from build123d import *

# Parameters (mm, degrees)
SKETCH_1_W          = 8
SKETCH_1_H          = 5
EXTRUDE_1_DEPTH     = 4
SKETCH_2_W          = 2
SKETCH_2_H          = 5
CUT_EXTRUDE_1_DEPTH = 3
SKETCH_3_R          = 1.65
CUT_EXTRUDE_2_DEPTH = 5


with BuildPart() as part:
    # Эскиз1 → Бобышка-Вытянуть1 (new body)
    with BuildSketch(Plane.XY):
        Rectangle(SKETCH_1_W, SKETCH_1_H)
    extrude(amount=EXTRUDE_1_DEPTH)

    # Эскиз2 → Вырез-Вытянуть1 (cut)
    with BuildSketch(Plane(origin=(4, 0, 0), x_dir=(0, 0, -1), z_dir=(1, 0, 0))):
        with Locations((-3, 0)):
            Rectangle(SKETCH_2_W, SKETCH_2_H)
    extrude(amount=-CUT_EXTRUDE_1_DEPTH, mode=Mode.SUBTRACT)

    # Эскиз3 → Вырез-Вытянуть2 (cut)
    with BuildSketch(Plane.XY.offset(4)):
        with Locations((-1.5, 0)):
            Circle(SKETCH_3_R)
    extrude(amount=-CUT_EXTRUDE_2_DEPTH, mode=Mode.SUBTRACT)


solid = part.part
Model file for the job. Use its own axes, mm. A direction names the side the tool comes from. Give positions to 0.01 mm unless a question says otherwise; leave off trailing zeros. Write each loop counter-clockwise with the first axis right and the second up, starting at its lowest first coordinate (ties: lowest second). Pieces come first, ordered by that corner, then holes. Notation, with made-up numbers: (49, -19) -> (79, -19) arc R27 cw to (79, 1) -> close; hole circle Ø8 at (-1, -10.75). An arc over 180 degrees is marked (long way). Write item = value, one per line.
(1) Mould opens along Y. For faces 3 (the face through (4, 0, 1)), 4 (the face through (0.074, 0.496, 2.028)), 5 (the face through (-1, -2.5, 2)), 6 (the face through (-1, 2.5, 2)) say: released by +Y, released by -Y, zero draft, split by the parting line, or undercut.
Determined:
face_3 = zero draft
face_4 = undercut
face_5 = released by -Y
face_6 = released by +Y
(2) Slice it at D-D, the plane y = -2.05. Give the cut face in (x, z), then the cut area to 3 significant figures.
Determined:
outline = (-4, 0) -> (4, 0) -> (4, 2) -> (1, 2) -> (1, 4) -> (-4, 4) -> close
area = 26.0 mm2
(3) Slice it at C-C, the plane z = 0.4. Give the cut face in (x, y), then the cut area to 3 significant figures.
Determined:
outline = (-4, -2.5) -> (4, -2.5) -> (4, 2.5) -> (-4, 2.5) -> close; hole circle Ø3.3 at (-1.5, 0)
area = 31.4 mm2
(4) Slice it at B-B, the plane x = -1.5. Give the cut face in (y, z).
Determined:
outline = (-2.5, 0) -> (-1.65, 0) -> (-1.65, 4) -> (-2.5, 4) -> close; (1.65, 0) -> (2.5, 0) -> (2.5, 4) -> (1.65, 4) -> close
(5) Probe line 1 along Y through (x, z) = (-1.5, 1.05); line 2 along Z through (x, y) = (3, 1.95); line 3 along X through (y, z) = (1, 1.3). List the from-to ranges inside material, lowest first.
Determined:
line_1 = -2.5 to -1.65, 1.65 to 2.5
line_2 = 0 to 2
line_3 = -4 to -2.81, -0.19 to 4
(6) Tool access for faces 1 (the face through (3, 0, 2)), 2 (the face through (-4, 0, 2)): list every direction of +Z, -Z, +X, -X, +Y, -Y with a clear straight run to the whole face (end or side of a thin tool).
Determined:
face_1 = +Z, +X, +Y, -Y
face_2 = +Z, -Z, -X, +Y, -Y
(7) Slice it at A-A, the plane y = 0. Give the cut face in (x, z), then the cut area to 3 significant figures.
Determined:
outline = (-4, 0) -> (-3.15, 0) -> (-3.15, 4) -> (-4, 4) -> close; (0.15, 0) -> (4, 0) -> (4, 2) -> (1, 2) -> (1, 4) -> (0.15, 4) -> close
area = 12.8 mm2
(8) Flat gauge pins, fed straight in: P1, Ø2, axis at x = 3, y = 0, coming from the -Z side; P2, Ø2.5, axis at x = -1.5, y = 0, coming from the -Z side. Where does each tip first touch, or does it go through?
Determined:
P1 = 0
P2 = through
